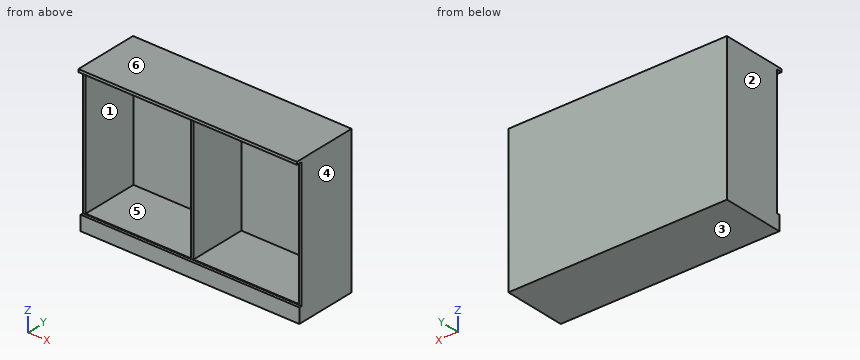
```python
from build123d import *

# Parameters (mm, degrees)
F0_W     = 19.05
F0_H     = 860.425
F1_DEPTH = 393.7
F2_W     = 1511.3
F2_H     = 884.555
F3_DEPTH = 19.05
F4_W     = 1511.3
F4_H     = 450.85
F5_DEPTH = 19.05
F6_W     = 1511.3
F6_H     = 431.8
F7_DEPTH = 101.6


with BuildPart() as f1:
    # F0 (on Front) → F1 (new body)
    with BuildSketch(Plane.XZ):
        Polygon((0, 879.475), (0, 860.425), (9.525, 860.425), (736.6, 860.425), (755.65, 860.425), (755.65, 879.475), align=None)
        Polygon((-9.525, 860.425), (0, 860.425), (0, 879.475), (-755.65, 879.475), (-755.65, 860.425), (-736.6, 860.425), align=None)
        with Locations((746.125, 430.2125)):
            Rectangle(F0_W, F0_H)
        Polygon((736.6, 0), (9.525, 0), (0, 0), (-9.525, 0), (-736.6, 0), (-755.65, 0), (-755.65, -5.08), (755.65, -5.08), (755.65, 0), align=None)
        with Locations((-746.125, 430.2125)):
            Rectangle(F0_W, F0_H)
        Polygon((9.525, 860.425), (0, 860.425), (-9.525, 860.425), (-9.525, 0), (0, 0), (9.525, 0), align=None)
    extrude(amount=F1_DEPTH)

    # F2 (on face) → F3 (join)
    with BuildSketch(Plane(origin=(0, 0, 0), x_dir=(-1, 0, 0), z_dir=(0, 1, 0))):
        with Locations((0, 437.1975)):
            Rectangle(F2_W, F2_H)
    extrude(amount=F3_DEPTH)

    # F4 (on face) → F5 (join)
    with BuildSketch(Plane.XY.offset(879.475)):
        with Locations((0, -206.375)):
            Rectangle(F4_W, F4_H)
    extrude(amount=F5_DEPTH)

    # F6 (on face) → F7 (join)
    with BuildSketch(Plane(origin=(0, 0, -5.08), x_dir=(1, 0, 0), z_dir=(0, 0, -1))):
        with Locations((0, 196.85)):
            Rectangle(F6_W, F6_H)
    extrude(amount=F7_DEPTH)


solid = f1.part
```
The model under review builds one solid part; all positions refer to its coordinate system, in mm. Face numbers are marked on the shaded views. A direction names the side the tool comes from. Round coordinates to 2 decimals unless told otherwise and drop trailing zeros. Order: outer loops, then holes, each group sorted by start corner. A loop starts at its lowest first (then second) coordinate and runs counter-clockwise, first axis right, second up. Notation, with made-up numbers: M 16,17 L 54,17 A20 cw 54,52 Z; hole C 0,60.25 d5. An arc over 180 degrees is marked long. Use a Markdown table: item, result.
1) Consider section B-B (y = -321). Write out the cut boundary in (x, z) (3 decimals).
Report:
| item | result |
|---|---|
| outline | M -755.65,-106.68 L 755.65,-106.68 L 755.65,898.525 L -755.65,898.525 Z; hole M -736.6,0 L -9.525,0 L -9.525,860.425 L -736.6,860.425 Z; hole M 9.525,0 L 736.6,0 L 736.6,860.425 L 9.525,860.425 Z |
2) Consider section C-C (z = 113). Write out the cut boundary in (x, y) (3 decimals).
Report:
| item | result |
|---|---|
| outline | M -755.65,-393.7 L -736.6,-393.7 L -736.6,0 L -9.525,0 L -9.525,-393.7 L 9.525,-393.7 L 9.525,0 L 736.6,0 L 736.6,-393.7 L 755.65,-393.7 L 755.65,19.05 L -755.65,19.05 Z |
3) Tool access review of the marked faces 5 and 6: name each direction out of +Z, -Z, +X, -X, +Y, -Y from which nothing blocks a thin tool from reaching the whole face with its end or side.
Report:
| item | result |
|---|---|
| face 5 | -Y |
| face 6 | +Z, +X, -X, +Y, -Y |
4) Wall thickness on line 1 along X through (y, z) = (-136, 226.5) (3 decimals); line 2 along Z through (x, y) = (-255, -220.5) (3 decimals); line 3 along Y through (x, z) = (654, 117.5): over which ranges is each line inside the solid? List them lowest first. Write a range as [from, to].
Report:
| item | result |
|---|---|
| line 1 | [-755.65, -736.6], [-9.525, 9.525], [736.6, 755.65] |
| line 2 | [-106.68, 0], [860.425, 898.525] |
| line 3 | [0, 19.05] |
5) Consider section A-A (x = -83). Write out the cut boundary in (y, z) (3 decimals).
Report:
| item | result |
|---|---|
| outline | M -431.8,879.475 L -393.7,879.475 L -393.7,860.425 L 0,860.425 L 0,0 L -393.7,0 L -393.7,-5.08 L -412.75,-5.08 L -412.75,-106.68 L 19.05,-106.68 L 19.05,898.525 L -431.8,898.525 Z |
6) Draft analysis for pull direction X (two halves, no side actions). For the marked faces 1, 2, 3 and 4, state which applies: released by +X, released by -X, zero draft, split by the parting line, or undercut.
Report:
| item | result |
|---|---|
| face 1 | undercut |
| face 2 | released by -X |
| face 3 | zero draft |
| face 4 | released by +X |
